```python
from build123d import *

# Parameters (mm, degrees)
IZIM1_W                     = 48
IZIM1_H                     = 46.07
Y_KSEKLIK_EKSTR_ZYON1_DEPTH = 3
IZIM2_W                     = 4
IZIM2_H                     = 46.07
Y_KSEKLIK_EKSTR_ZYON2_DEPTH = 50
IZIM3_W                     = 4
IZIM3_H                     = 46.07
Y_KSEKLIK_EKSTR_ZYON3_DEPTH = 7


with BuildPart() as part:
    # Çizim1 → Yükseklik-Ekstrüzyon1 (new body)
    with BuildSketch(Plane(origin=(0, 0, 0), x_dir=(1, 0, 0), z_dir=(0, 1, 0))):
        Rectangle(IZIM1_W, IZIM1_H)
    y_kseklik_ekstr_zyon1 = extrude(amount=Y_KSEKLIK_EKSTR_ZYON1_DEPTH)

    # Çizim2 → Yükseklik-Ekstrüzyon2 (add)
    with BuildSketch(Plane(origin=(0, 3, 0), x_dir=(1, 0, 0), z_dir=(0, 1, 0))):
        Rectangle(IZIM2_W, IZIM2_H)
    extrude(amount=Y_KSEKLIK_EKSTR_ZYON2_DEPTH)

    # Aynalama1: Yükseklik-Ekstrüzyon1 across plane
    add(y_kseklik_ekstr_zyon1.mirror(Plane.ZX.offset(26.5)))

    # Çizim3 → Yükseklik-Ekstrüzyon3 (add)
    with BuildSketch(Plane(origin=(0, 53, 0), x_dir=(1, 0, 0), z_dir=(0, 1, 0))):
        with Locations((22, 0)):
            Rectangle(IZIM3_W, IZIM3_H)
    y_kseklik_ekstr_zyon3 = extrude(amount=Y_KSEKLIK_EKSTR_ZYON3_DEPTH)

    # Aynalama2: Yükseklik-Ekstrüzyon3 across plane
    add(y_kseklik_ekstr_zyon3.mirror(Plane(origin=(0, 0, 0), x_dir=(0, 0, 1), z_dir=(1, 0, 0))))


solid = part.part
```
Can you work these out from the model? Positions are in its coordinate system, mm. A direction names the side the tool comes from. Round coordinates to 2 decimals unless told otherwise and drop trailing zeros. Loops run counter-clockwise (first coordinate to the right, second up) from the corner with the lowest first, then second, coordinate; pieces in that order, holes last. Notation, with made-up numbers: (8.5, -28.5) -> (33.5, -28.5) arc R27 ccw to (33.5, 6.5) -> close; hole circle Ø8 at (81, 70). An arc over 180 degrees is marked (long way). One line per item, written item: value. Start each with the question number.
1. If we section it at B-B, the plane y = 54: Write out the boundary of the cut face in (x, z) (3 decimals).
2. For pin 1 (6.5 mm diameter, centred on x = 14.5, z = 7.5, fed in from +Y); pin 2 (23 mm diameter, centred on y = 33, z = -7, fed in from +X); pin 3 (2 mm diameter, centred on y = 45, z = 9.5, fed in from -X), each with a flat end and sliding along its axis, tell me the tip position at first contact or that it passes through.
3. If we section it at C-C, the plane z = -18: Write out the boundary of the cut face in (x, y).
4. If we section it at D-D, the plane y = 7: Write out the boundary of the cut face in (x, z) (3 decimals), then the cut area to 3 significant figures.
5. If we mould it in two halves opening along Y, with no side actions, what happens to faces 5 (the flat face through (-2, 26, 0)), 6 (the flat face through (0, 53, 0)), 7 (the flat face through (0, 30, 23.035))? For each: pulls with the +Y half, pulls with the -Y half, needs draft (parallel to the pull), parting line crosses it, or undercut.
6. If I drill on probe 1 along Y at (x, z) = (-15.5, 21); probe 2 along X at (y, z) = (58, 18.5); probe 3 along X at (y, z) = (4, -19), over which ranges is the centre line in solid material (lowest first)?
7. For faces 1 (the flat face through (20, 56, 0)), 2 (the flat face through (0, 0, 0)), 3 (the flat face through (-13, 50, 0)), 4 (the flat face through (13, 50, 0)), which set-ups out of +Z, -Z, +X, -X, +Y, -Y let a thin tool reach every point of the face, with its end or its side?
8. If we section it at A-A, the plane x = -18: Write out the boundary of the cut face in (y, z) (3 decimals), then the cut area to 3 significant figures.
Calculated:
1. outline: (-24, -23.035) -> (-20, -23.035) -> (-20, 23.035) -> (-24, 23.035) -> close; (20, -23.035) -> (24, -23.035) -> (24, 23.035) -> (20, 23.035) -> close
2. pin 1: stops at y = 53
2. pin 2: stops at x = 2
2. pin 3: stops at x = -2
3. outline: (-24, 0) -> (24, 0) -> (24, 3) -> (2, 3) -> (2, 50) -> (24, 50) -> (24, 60) -> (20, 60) -> (20, 53) -> (-20, 53) -> (-20, 60) -> (-24, 60) -> (-24, 50) -> (-2, 50) -> (-2, 3) -> (-24, 3) -> close
4. outline: (-2, -23.035) -> (2, -23.035) -> (2, 23.035) -> (-2, 23.035) -> close
4. area: 184 mm²
5. face 5: undercut
5. face 6: pulls with the +Y half
5. face 7: needs draft
6. probe 1: y = 0 to 3, 50 to 53
6. probe 2: x = -24 to -20, 20 to 24
6. probe 3: x = -2 to 2
7. face 1: +Z, -Z, +Y
7. face 2: +Z, -Z, +X, -X, -Y
7. face 3: +Z, -Z, -X
7. face 4: +Z, -Z, +X
8. outline: (0, -23.035) -> (3, -23.035) -> (3, 23.035) -> (0, 23.035) -> close; (50, -23.035) -> (53, -23.035) -> (53, 23.035) -> (50, 23.035) -> close
8. area: 276 mm²
